Could you check a few things on this model? Use its own coordinates, in mm. A direction names the side the tool comes from. Coordinates: 2 decimals unless noted, no trailing zeros. Loops run counter-clockwise (first coordinate to the right, second up) from the corner with the lowest first, then second, coordinate; pieces in that order, holes last.
from build123d import *

# Parameters (mm, degrees)
SKETCH1_R          = 24
EXTRUDE1_DEPTH     = 5
SKETCH2_R          = 6.5
EXTRUDE2_DEPTH     = 7
SKETCH3_R          = 29
SKETCH3_R_2        = 24
EXTRUDE3_DEPTH     = 7
CUT_EXTRUDE1_DEPTH = 0.6


with BuildPart() as part:
    # Sketch1 → Extrude1 (new body)
    with BuildSketch(Plane.XY):
        Circle(SKETCH1_R)
    extrude(amount=EXTRUDE1_DEPTH)

    # Sketch2 → Extrude2 (add)
    with BuildSketch(Plane.XY.offset(5)):
        Circle(SKETCH2_R)
    extrude(amount=EXTRUDE2_DEPTH)

    # Sketch3 → Extrude3 (add)
    with BuildSketch(Plane(origin=(0, 0, 0), x_dir=(-1, 0, 0), z_dir=(0, 0, -1))):
        Circle(SKETCH3_R)
        Circle(SKETCH3_R_2, mode=Mode.SUBTRACT)
    extrude(amount=-EXTRUDE3_DEPTH)

    # Sketch4 → Cut-Extrude1 (cut)
    with BuildSketch(Plane.XY.offset(7)):
        with BuildLine():
            Line((3.39411255, 23.758787848), (4.101219331, 28.708535316))
            ThreePointArc((4.101219331, 28.708535316), (2.055781583, 28.927042056), (0, 29))
            ThreePointArc((0, 29), (-2.055781583, 28.927042056), (-4.101219331, 28.708535316))
            Line((-4.101219331, 28.708535316), (-3.39411255, 23.758787848))
            ThreePointArc((-3.39411255, 23.758787848), (-1.701336482, 23.939621012), (0, 24))
            ThreePointArc((0, 24), (1.701336482, 23.939621012), (3.39411255, 23.758787848))
        make_face()
        with BuildLine():
            Line((23.758787848, -3.39411255), (28.708535316, -4.101219331))
            ThreePointArc((28.708535316, -4.101219331), (28.927042056, -2.055781583), (29, 0))
            ThreePointArc((29, 0), (28.927042056, 2.055781583), (28.708535316, 4.101219331))
            Line((28.708535316, 4.101219331), (23.758787848, 3.39411255))
            ThreePointArc((23.758787848, 3.39411255), (23.939621012, 1.701336482), (24, 0))
            ThreePointArc((24, 0), (23.939621012, -1.701336482), (23.758787848, -3.39411255))
        make_face()
        with BuildLine():
            Line((3.39411255, -23.758787848), (4.101219331, -28.708535316))
            ThreePointArc((4.101219331, -28.708535316), (2.055781583, -28.927042056), (0, -29))
            ThreePointArc((0, -29), (-2.055781583, -28.927042056), (-4.101219331, -28.708535316))
            Line((-4.101219331, -28.708535316), (-3.39411255, -23.758787848))
            ThreePointArc((-3.39411255, -23.758787848), (-1.701336482, -23.939621012), (0, -24))
            ThreePointArc((0, -24), (1.701336482, -23.939621012), (3.39411255, -23.758787848))
        make_face()
        with BuildLine():
            Line((-23.758787848, -3.39411255), (-28.708535316, -4.101219331))
            ThreePointArc((-28.708535316, -4.101219331), (-28.927042056, -2.055781583), (-29, 0))
            ThreePointArc((-29, 0), (-28.927042056, 2.055781583), (-28.708535316, 4.101219331))
            Line((-28.708535316, 4.101219331), (-23.758787848, 3.39411255))
            ThreePointArc((-23.758787848, 3.39411255), (-23.939621012, 1.701336482), (-24, 0))
            ThreePointArc((-24, 0), (-23.939621012, -1.701336482), (-23.758787848, -3.39411255))
        make_face()
    extrude(amount=-CUT_EXTRUDE1_DEPTH, mode=Mode.SUBTRACT)


solid = part.part
(1) We'd pull the mould along X, two halves only. Please class faces 1 (the face through (-18, 18, 7)), 2 (the face through (-22.17, -9.19, 5.99)), 3 (the face through (-26.789, -11.107, 3.451)): +X half, -X half, draft (parallel to the pull), parting line (faces both ways), or undercut.
Answers:
face 1: draft
face 2: undercut
face 3: parting line
(2) I need wall thicknesses on probe 1 along Y at (x, z) = (0, 5.9); probe 2 along Z at (x, y) = (-20, -13.5); probe 3 along Z at (x, y) = (-4, 16.5). Which ranges of each line are inside material? Lowest first, please.
Answers:
probe 1: y = -29 to -24, -6.5 to 6.5, 24 to 29
probe 2: z = 0 to 7
probe 3: z = 0 to 5
(3) Imagine slicing it at D-D, the plane y = -7.5. Write out the boundary of the cut face in (x, z).
Answers:
outline: (-28.01, 0) - (28.01, 0) - (28.01, 7) - (22.8, 7) - (22.8, 5) - (-22.8, 5) - (-22.8, 7) - (-28.01, 7) - close
(4) Imagine slicing it at A-A, the plane y = 0. Write out the boundary of the cut face in (x, z).
Answers:
outline: (-29, 0) - (29, 0) - (29, 6.4) - (24, 6.4) - (24, 5) - (6.5, 5) - (6.5, 12) - (-6.5, 12) - (-6.5, 5) - (-24, 5) - (-24, 6.4) - (-29, 6.4) - close
(5) Which directions (+Z, -Z, +X, -X, +Y, -Y) give clear straight access to the entire face, cutting with the end or side of a thin tool? Please do faces 4 (the face through (-26, 0, 6.4)), 5 (the face through (26, 0, 6.4)), 6 (the face through (-5.158, -3.955, 8.451)), 7 (the face through (0, 26, 6.4)), 8 (the face through (0, -26, 6.4)).
Answers:
face 4: +Z, -X
face 5: +Z, +X
face 6: +Z
face 7: +Z, +Y
face 8: +Z, -Y
(6) For pin 1 (2.5 mm diameter, centred on x = -0.5, y = 27, fed in from +Z); pin 2 (1.5 mm diameter, centred on x = 19, z = 7.5, fed in from +Y); pin 3 (6 mm diameter, centred on x = 14, z = 8.5, fed in from -Y); pin 4 (1.5 mm diameter, centred on y = -19.5, z = 8, fed in from +X), each with a flat end and sliding along its axis, tell me the tip position at first contact or that it passes through.
Answers:
pin 1: stops at z = 6.4
pin 2: stops at y = 22.38
pin 3: stops at y = -26.66
pin 4: passes through
(7) Imagine slicing it at C-C, the plane z = 2.75. Write out the boundary of the cut face in (x, y), and give its area (3 significant figures).
Answers:
outline: circle Ø58 at (0, 0)
area: 2,640 mm2
